The listing builds one solid part. Answer for the finished solid, in the listing's coordinates (mm). A direction names the side the tool comes from. Coordinates: 2 decimals unless noted, no trailing zeros. Order: outer loops, then holes, each group sorted by start corner. A loop starts at its lowest first (then second) coordinate and runs counter-clockwise, first axis right, second up.
```python
from build123d import *

# Parameters (mm, degrees)
BOSS_EXTRUDE1_DEPTH = 116
CUT_EXTRUDE1_REACH  = 13
SKETCH3_R           = 1.65
SKETCH4_R           = 3
CUT_EXTRUDE2_DEPTH  = 4
FILLET1_R           = 1


with BuildPart() as part:
    # Sketch2 → Boss-Extrude1 (new body)
    with BuildSketch(Plane(origin=(0, 0, 0), x_dir=(0, 0, -1), z_dir=(1, 0, 0))):
        Polygon((0, 0), (0, 12), (-5, 12), (-5, 16), (6, 16), (6, 0), align=None)
    extrude(amount=BOSS_EXTRUDE1_DEPTH)

    # Sketch3 → Cut-Extrude1 (cut, up to next)
    with BuildSketch(Plane(origin=(0, 0, -6), x_dir=(-1, 0, 0), z_dir=(0, 0, -1)), mode=Mode.PRIVATE) as cut_extrude1_sk1:
        with Locations((-103, 5)):
            Circle(SKETCH3_R)
    cut_extrude1_tool1 = extrude(cut_extrude1_sk1.sketch, amount=-CUT_EXTRUDE1_REACH, mode=Mode.PRIVATE) & part.part
    add(cut_extrude1_tool1.solids().sort_by_distance((103, 5, -6))[0], mode=Mode.SUBTRACT)
    # Sketch3 → Cut-Extrude1 (cut, up to next)
    with BuildSketch(Plane(origin=(0, 0, -6), x_dir=(-1, 0, 0), z_dir=(0, 0, -1)), mode=Mode.PRIVATE) as cut_extrude1_sk2:
        with Locations((-13, 5)):
            Circle(SKETCH3_R)
    cut_extrude1_tool2 = extrude(cut_extrude1_sk2.sketch, amount=-CUT_EXTRUDE1_REACH, mode=Mode.PRIVATE) & part.part
    add(cut_extrude1_tool2.solids().sort_by_distance((13, 5, -6))[0], mode=Mode.SUBTRACT)
    # Sketch3 → Cut-Extrude1 (cut, up to next)
    with BuildSketch(Plane(origin=(0, 0, -6), x_dir=(-1, 0, 0), z_dir=(0, 0, -1)), mode=Mode.PRIVATE) as cut_extrude1_sk3:
        with Locations((-58, 5)):
            Circle(SKETCH3_R)
    cut_extrude1_tool3 = extrude(cut_extrude1_sk3.sketch, amount=-CUT_EXTRUDE1_REACH, mode=Mode.PRIVATE) & part.part
    add(cut_extrude1_tool3.solids().sort_by_distance((58, 5, -6))[0], mode=Mode.SUBTRACT)

    # Sketch4 → Cut-Extrude2 (cut)
    with BuildSketch(Plane(origin=(0, 0, -6), x_dir=(-1, 0, 0), z_dir=(0, 0, -1))):
        with Locations((-103, 5)):
            Circle(SKETCH4_R)
        with Locations((-58, 5)):
            Circle(SKETCH4_R)
        with Locations((-13, 5)):
            Circle(SKETCH4_R)
    extrude(amount=-CUT_EXTRUDE2_DEPTH, mode=Mode.SUBTRACT)

    # Fillet1
    fillet1_edges = [part.edges().sort_by_distance(p)[0] for p in [
        (58, 0, 0),
        (58, 12, 5),
        (58, 16, 5),
        (58, 16, -6),
        (58, 0, -6),
    ]]
    fillet(fillet1_edges, radius=FILLET1_R)


solid = part.part
```
1) For faces 1 (the cylindrical face through (105.4, 3.2, -4)), 2 (the flat face through (57, 8, 0)), 3 (the cylindrical face through (59.65, 5.07, -1.01)), determine the directions among +Z, -Z, +X, -X, +Y, -Y from which every point of the face is accessible in a straight line to the end or side of a thin tool.
2) A cutting plane is placed at A-A, the plane x = 103. Write down the section's boundary in (y, z), plus the area to 3 significant figures.
3) Straight lines are drawn through the part: probe 1 along Y at (x, z) = (13, -3.2); probe 2 along X at (y, z) = (6, -2.25); probe 3 along Z at (x, y) = (52, 9.5). For each, find the intervals that lie inside material, in ascending order.
4) A cutting plane is placed at B-B, the plane y = 5. Write down the section's boundary in (x, z), plus the area to 3 significant figures.
5) A cutting plane is placed at C-C, the plane x = 41.5. Write down the section's boundary in (y, z).
6) The mould has two halves that part along X. Classify faces 4 (the flat face through (57, 14, 5)), 5 (the flat face through (116, 10, -2)), 6 (the cylindrical face through (104.65, 5.07, -1.01)): released by +X, released by -X, zero draft, split by the parting line, or undercut.
7) Each of these flat-tipped pins is pushed along its axis until it touches: P1, Ø9, axis at x = 84, y = 6.5, coming from the +Z side; P2, Ø5, axis at x = 13, y = 6.5, coming from the -Z side; P3, Ø4.5, axis at x = 81, z = 1.5, coming from the -Y side; P4, Ø1.8, axis at x = 102.5, y = 3.5, coming from the -Z side. Where does it stop, or does it pass through?
Working result:
1. face 1: -Z
1. face 2: +Z, +X, -X, -Y
1. face 3: +Z, -Z
2. outline: (0, -5) arc R1 ccw to (1, -6) - (2, -6) - (2, -2) - (3.35, -2) - (3.35, 0) - (1, 0) arc R1 ccw to (0, -1) - close; (6.65, -2) - (8, -2) - (8, -6) - (15, -6) arc R1 ccw to (16, -5) - (16, 4) arc R1 ccw to (15, 5) - (13, 5) arc R1 ccw to (12, 4) - (12, 0) - (6.65, 0) - close
2. area: 84.3 mm2
3. probe 1: y = 0 to 2, 8 to 16
3. probe 2: x = 0 to 10.17, 15.83 to 55.17, 60.83 to 100.17, 105.83 to 116
3. probe 3: z = -6 to 0
4. outline: (0, -6) - (10, -6) - (10, -2) - (11.35, -2) - (11.35, 0) - (0, 0) - close; (14.65, -2) - (16, -2) - (16, -6) - (55, -6) - (55, -2) - (56.35, -2) - (56.35, 0) - (14.65, 0) - close; (59.65, -2) - (61, -2) - (61, -6) - (100, -6) - (100, -2) - (101.35, -2) - (101.35, 0) - (59.65, 0) - close; (104.65, -2) - (106, -2) - (106, -6) - (116, -6) - (116, 0) - (104.65, 0) - close
4. area: 604 mm2
5. outline: (0, -5) arc R1 ccw to (1, -6) - (15, -6) arc R1 ccw to (16, -5) - (16, 4) arc R1 ccw to (15, 5) - (13, 5) arc R1 ccw to (12, 4) - (12, 0) - (1, 0) arc R1 ccw to (0, -1) - close
6. face 4: zero draft
6. face 5: released by +X
6. face 6: undercut
7. P1: stops at z = 0
7. P2: stops at z = -6
7. P3: stops at y = 0.03
7. P4: stops at z = -2
